Can you work these out from the model? Positions are in its coordinate system, mm. A direction names the side the tool comes from. Give positions to 0.01 mm unless a question says otherwise; leave off trailing zeros. Write each loop counter-clockwise with the first axis right and the second up, starting at its lowest first coordinate (ties: lowest second). Pieces come first, ordered by that corner, then holes. Notation, with made-up numbers: (78, -20.5) - (107, -20.5) arc R17 cw to (107, -15.5) - close; hole circle Ø6 at (-18, 73.25). An arc over 180 degrees is marked (long way). Use a Markdown table: item, result. Add a question column.
```python
from build123d import *

# Parameters (mm, degrees)
CROQUIS1_W                      = 275
CROQUIS1_H                      = 260
BRIDA_BASE1_DEPTH               = 6
CORTAR_EXTRUIR1_DEPTH           = 190.320495457
CORTAR_EXTRUIR1_DEPTH_BACK      = 190.320495457
CROQUIS3_R                      = 1.875
CORTAR_EXTRUIR2_DEPTH           = 190.320495457
CORTAR_EXTRUIR2_DEPTH_BACK      = 190.320495457
RANURA_START                    = -6
RANURA_DE_MARGEN_PARA_M61_DEPTH = 6
CROQUIS9_R                      = 1.2
CORTAR_EXTRUIR4_DEPTH           = 190.320495457
TALADRO_DE_MARGEN_PARA_M31_D    = 3.4


# Read off the part's stored shape, not the designer's step: Ranura de margen para M61
# Sheet-metal steps are written as plain solids
with BuildPart() as part:
    # Croquis1 → Brida base1 (new body)
    with BuildSketch(Plane.XY):
        Rectangle(CROQUIS1_W, CROQUIS1_H)
    extrude(amount=-BRIDA_BASE1_DEPTH)

    # Croquis3 → Cortar-Extruir1 (cut, two sides: drawn at the far end of the back side and taken through both)
    with BuildSketch(Plane(origin=(0, 0, -6), x_dir=(-1, 0, 0), z_dir=(0, 0, -1)).offset(-CORTAR_EXTRUIR1_DEPTH_BACK)):
        with Locations((-88, 84.63)):
            Circle(CROQUIS3_R)
        with Locations((-60, 124.63)):
            Circle(CROQUIS3_R)
        with Locations((-88, 124.63)):
            Circle(CROQUIS3_R)
        with Locations((-88, 62.63)):
            Circle(CROQUIS3_R)
        with Locations((-88, 43.63)):
            Circle(CROQUIS3_R)
    extrude(amount=CORTAR_EXTRUIR1_DEPTH + CORTAR_EXTRUIR1_DEPTH_BACK, mode=Mode.SUBTRACT)

    # Croquis4 → Cortar-Extruir2 (cut, two sides: drawn at the far end of the back side and taken through both)
    with BuildSketch(Plane.XY.offset(-CORTAR_EXTRUIR2_DEPTH_BACK)):
        with BuildLine():
            Line((-101.5, 38.67), (29.25, 38.67))
            ThreePointArc((29.25, 38.67), (41.25, 50.67), (29.25, 62.67))
            Line((29.25, 62.67), (-101.5, 62.67))
            ThreePointArc((-101.5, 62.67), (-113.5, 50.67), (-101.5, 38.67))
        make_face()
    extrude(amount=CORTAR_EXTRUIR2_DEPTH + CORTAR_EXTRUIR2_DEPTH_BACK, mode=Mode.SUBTRACT)

    # Ranura de margen para M61 outline → Ranura de margen para M61 (cut)
    with BuildSketch(Plane.XY.offset(RANURA_START)):
        with BuildLine():
            Line((117, 118), (120, 118))
            ThreePointArc((120, 118), (123.5, 121.5), (120, 125))
            Line((120, 125), (117, 125))
            ThreePointArc((117, 125), (113.5, 121.5), (117, 118))
        make_face()
        with BuildLine():
            ThreePointArc((-117, 118), (-113.5, 121.5), (-117, 125))
            Line((-117, 125), (-120, 125))
            ThreePointArc((-120, 125), (-123.5, 121.5), (-120, 118))
            Line((-120, 118), (-117, 118))
        make_face()
        with BuildLine():
            Line((-120, -125), (-117, -125))
            ThreePointArc((-117, -125), (-113.5, -121.5), (-117, -118))
            Line((-117, -118), (-120, -118))
            ThreePointArc((-120, -118), (-123.5, -121.5), (-120, -125))
        make_face()
        with BuildLine():
            ThreePointArc((120, -125), (123.5, -121.5), (120, -118))
            Line((120, -118), (117, -118))
            ThreePointArc((117, -118), (113.5, -121.5), (117, -125))
            Line((117, -125), (120, -125))
        make_face()
    extrude(amount=RANURA_DE_MARGEN_PARA_M61_DEPTH, mode=Mode.SUBTRACT)

    # Croquis9 → Cortar-Extruir4 (cut, through all)
    with BuildSketch(Plane.XY):
        with Locations((5, -127.5)):
            Circle(CROQUIS9_R)
    extrude(amount=-CORTAR_EXTRUIR4_DEPTH, mode=Mode.SUBTRACT)

    # Taladro de margen para M31 (through all)
    with Locations(Plane.XY):
        with Locations((10, 125), (-10, 125)):
            Hole(TALADRO_DE_MARGEN_PARA_M31_D / 2)


solid = part.part
```
Q1. Suppose I cut it at A-A (z = -0.9). Give the number of separate pieces and of enclosed holes in the cut face, and give its area (3 significant figures).
Q2. I'm going to push a flat-ended pin straight in: P1, Ø2.5, axis at x = 10, y = 125, coming from the +Z side. Where does the tip first touch, or does it pass through?
Q3. If I drill on probe 1 along Y at (x, z) = (88, -4.1) (3 decimals); probe 2 along Y at (x, z) = (118.5, -2.7); probe 3 along Y at (x, z) = (-10, -2.6), over which ranges is the centre line in solid material (lowest first)? Write a range as [from, to].
Q4. Suppose I cut it at B-B (x = -18). Please give me the cut outline in (y, z).
Q5. If we mould it in two halves opening along X, with no side actions, what happens to faces 3 (the flat face through (-37, 38.67, -3)), 4 (the flat face through (-2, 2, -6)), 5 (the flat face through (137.5, -2, -3))? For each: released by +X, released by -X, zero draft, split by the parting line, or undercut.
Q6. On a 3-axis mill with a long thin cutter (end or side, diameter ignored), from which of +Z, -Z, +X, -X, +Y, -Y can I reach the whole of each face in a straight line? I mean faces 1 (the flat face through (-2, 130, -3)), 2 (the cylindrical face through (-113.5, -121.6, -3)). Say none if no direction works.
Derived:
| question | item | result |
|---|---|---|
| 1 | separate pieces | 1 |
| 1 | enclosed holes | 13 |
| 1 | area | 67,600 mm² |
| 2 | P1 | through |
| 3 | probe 1 | [-130, 41.755], [45.505, 60.755], [64.505, 82.755], [86.505, 122.755], [126.505, 130] |
| 3 | probe 2 | [-130, -125], [-118, 118], [125, 130] |
| 3 | probe 3 | [-130, 38.67], [62.67, 123.3], [126.7, 130] |
| 4 | outline | (-130, -6) - (38.67, -6) - (38.67, 0) - (-130, 0) - close; (62.67, -6) - (130, -6) - (130, 0) - (62.67, 0) - close |
| 5 | face 3 | undercut |
| 5 | face 4 | zero draft |
| 5 | face 5 | released by +X |
| 6 | face 1 | +Z, -Z, +X, -X, +Y |
| 6 | face 2 | +Z, -Z |
